Verification items for the finished model (mm, model axes). Give positions to 0.01 mm unless a question says otherwise; leave off trailing zeros. Order: outer loops, then holes, each group sorted by start corner. A loop starts at its lowest first (then second) coordinate and runs counter-clockwise, first axis right, second up. Notation, with made-up numbers: (10, 7) - (18, 7) arc R30 cw to (18, 30) - close; hole circle Ø6 at (79.5, -7). An arc over 180 degrees is marked (long way). Answer as a JSON object with one key per item and string values.
```python
from build123d import *

# Parameters (mm, degrees)
SKETCH1_R           = 2.125
BOSS_EXTRUDE1_DEPTH = 4.7625
FILLET1_R           = 6.35
FILLET2_R           = 6.35
SKETCH3_W           = 63.5
SKETCH3_H           = 50.8
BOSS_EXTRUDE2_DEPTH = 4.7625
FILLET3_R           = 76.2
SKETCH8_R           = 2.125
CUT_EXTRUDE3_DEPTH  = 19.05
SKETCH10_R          = 2
CUT_EXTRUDE7_DEPTH  = 335.215390296


with BuildPart() as part:
    # Sketch1 → Boss-Extrude1 (new body)
    with BuildSketch(Plane.XY):
        with BuildLine():
            Line((0, 0), (0, -76.2))
            ThreePointArc((0, -76.2), (152.4, -108.007732044), (304.8, -76.2))
            Line((304.8, -76.2), (304.8, 0))
            ThreePointArc((304.8, 0), (152.4, -86.218997603), (0, 0))
        make_face()
        with Locations(Location((19.05, -57.207732044, 0), (0, 0, 180))):
            Circle(SKETCH1_R, mode=Mode.SUBTRACT)
        with Locations(Location((285.75, -57.207732044, 0), (0, 0, 180))):
            Circle(SKETCH1_R, mode=Mode.SUBTRACT)
    extrude(amount=BOSS_EXTRUDE1_DEPTH)

    # Fillet1
    fillet1_edges = [part.edges().sort_by_distance(p)[0] for p in [
        (304.8, 0, 2.38125),
        (0, 0, 2.38125),
    ]]
    fillet(fillet1_edges, radius=FILLET1_R)

    # Fillet2
    fillet2_edges = [part.edges().sort_by_distance(p)[0] for p in [
        (304.8, -76.2, 2.38125),
        (0, -76.2, 2.38125),
    ]]
    fillet(fillet2_edges, radius=FILLET2_R)

    # Sketch3 → Boss-Extrude2 (add)
    with BuildSketch(Plane.XY.offset(4.7625)):
        with Locations((152.4, -111.618997603)):
            Rectangle(SKETCH3_W, SKETCH3_H)
    extrude(amount=-BOSS_EXTRUDE2_DEPTH)

    # Fillet3
    # the kernel refuses this fillet: 76.2 mm, written as the material it adds along each edge
    with BuildSketch(Plane(origin=(184.15, -106.682510638, 4.7625), x_dir=(0.9886965633546299, 0.14993033585883936, 0), z_dir=(0, 0, -1))) as fillet3_piece_1:
        with BuildLine():
            CenterArc((56.174032607, 76.02868739), FILLET3_R, 217.166641645, 48.990660759)
            Line((-4.548359679, 29.993580407), (-5.762807525, 29.072878267))
            ThreePointArc((-5.762807525, 29.072878267), (-3.780953402, 14.768296372), (-1.506773563, -0.228493832))
            Line((-1.506773563, -0.228493832), (0.102134605, -1.520573748))
            ThreePointArc((0.102134605, -1.520573748), (25.533651185, -0.667436951), (50.965167766, -1.520573748))
            Line((50.965167766, -1.520573748), (51.06730237, 0))
        make_face()
    extrude(amount=4.7625)
    with BuildSketch(Plane(origin=(120.65, -106.682510638, 4.7625), x_dir=(0, -1, 0), z_dir=(0, 0, -1))) as fillet3_piece_2:
        with BuildLine():
            CenterArc((66.747110364, 66.938079624), FILLET3_R, 192.465587038, 48.990660759)
            Line((-7.656537796, 50.490066353), (-9.144610759, 50.161106088))
            ThreePointArc((-9.144610759, 50.161106088), (-4.488161518, 25.14496413), (-1.518699114, -0.127))
            Line((-1.518699114, -0.127), (0, -1.524))
            ThreePointArc((0, -1.524), (15.168243483, -1.524), (29.608274497, -1.338761592))
            Line((29.608274497, -1.338761592), (30.336486965, 0))
        make_face()
    extrude(amount=4.7625)

    # Sketch8 → Cut-Extrude3 (cut)
    with BuildSketch(Plane(origin=(0, 0, 0), x_dir=(-1, 0, 0), z_dir=(0, 0, -1))):
        with Locations((-171.45, -125.902330937)):
            Circle(SKETCH8_R)
        with Locations((-133.35, -125.902330937)):
            Circle(SKETCH8_R)
    extrude(amount=-CUT_EXTRUDE3_DEPTH, mode=Mode.SUBTRACT)

    # Sketch10 → Cut-Extrude7 (cut, through all)
    with BuildSketch(Plane.XY.offset(4.7625)):
        with Locations((133.35, -102.618997603)):
            Circle(SKETCH10_R)
        with Locations((171.45, -102.618997603)):
            Circle(SKETCH10_R)
    extrude(amount=-CUT_EXTRUDE7_DEPTH, mode=Mode.SUBTRACT)


solid = part.part
```
(1) Section check C-C (x = 77.5). Record the cut outline in (y, z).
Computed values:
{"outline": "(-101.04, 0) - (-69.67, 0) - (-69.67, 4.76) - (-101.04, 4.76) - close"}
(2) Gauge pin test, flat end, axial feed: pin 1 Ø3.5 at (x, y) = (133.35, -102.62) entering from +Z. Record the tip position at first contact, or that the pin passes through.
Computed values:
{"pin 1": "passes through"}
(3) Section check D-D (y = -109). Record the cut outline in (x, z).
Computed values:
{"outline": "(94.4, 0) - (210.4, 0) - (210.4, 4.76) - (94.4, 4.76) - close"}
(4) Material ranges on line 1 along Y through (x, z) = (133.35, 1.3); line 2 along X through (y, z) = (-58.5, 1.3); line 3 along X through (y, z) = (-65.5, 1.8), recorded low to high. Write a range as [from, to].
Computed values:
{"line 1": "y = [-137.02, -128.03], [-123.78, -104.62], [-100.62, -85.2]", "line 2": "x = [0, 17.36], [20.74, 57.07], [247.73, 284.06], [287.44, 304.8]", "line 3": "x = [0, 69.1], [235.7, 304.8]"}
(5) Release check for a two-part mould opening along X. For faces 1 (the cylindrical face through (267.8, -90.11, 2.35)), 2 (the flat face through (150, -90, 0)), 3 (the cylindrical face through (36.069, -89.813, 2.348)), 4 (the cylindrical face through (4.203, -14.606, 2.415)) record: pulls with the +X half, pulls with the -X half, needs draft (parallel to the pull), parting line crosses it, or undercut.
Computed values:
{"face 1": "pulls with the +X half", "face 2": "needs draft", "face 3": "pulls with the -X half", "face 4": "undercut"}
(6) Section check A-A (y = -24.5). Record the cut outline in (x, z).
Computed values:
{"outline": "(0, 0) - (17.72, 0) - (17.72, 4.76) - (0, 4.76) - close; (287.08, 0) - (304.8, 0) - (304.8, 4.76) - (287.08, 4.76) - close"}
(7) Section check B-B (z = 3.4). Record the cut outline in (x, y) (3 decimals), then the cut area to 3 significant figures.
Computed values:
{"outline": "(0, -72.018) arc R6.35 ccw to (3.875, -77.866) arc R381 ccw to (70.16, -99.026) arc R76.2 cw to (120.65, -137.019) - (184.15, -137.019) arc R76.2 cw to (234.64, -99.026) arc R381 ccw to (300.925, -77.866) arc R6.35 ccw to (304.8, -72.018) - (304.8, -20.582) arc R6.35 ccw to (293.414, -16.715) arc R177.8 cw to (11.386, -16.715) arc R6.35 ccw to (0, -20.582) - close; hole circle Ø4.25 at (19.05, -57.208); hole circle Ø4.25 at (133.35, -125.902); hole circle Ø4 at (133.35, -102.619); hole circle Ø4.25 at (171.45, -125.902); hole circle Ø4 at (171.45, -102.619); hole circle Ø4.25 at (285.75, -57.208)", "area": "13,700 mm²"}
